```python
from build123d import *

# Parameters (mm, degrees)
CROQUIS1_W              = 60
CROQUIS1_H              = 65
SALIENTE_EXTRUIR1_DEPTH = 80
CROQUIS2_R              = 12.5
CROQUIS2_R_2            = 2
CROQUIS2_R_3            = 4
CORTAR_EXTRUIR1_DEPTH   = 120.268604419
CROQUIS3_W              = 38
CROQUIS3_H              = 70
CORTAR_EXTRUIR4_DEPTH   = 50
CROQUIS4_W              = 8.5
CROQUIS4_H              = 70
CORTAR_EXTRUIR5_DEPTH   = 120.268604419
CROQUIS6_R              = 12.5
CROQUIS6_R_2            = 2
CORTAR_EXTRUIR6_DEPTH   = 120.268604419
CROQUIS15_R             = 11
SALIENTE_EXTRUIR6_DEPTH = 0.1
CROQUIS16_R             = 10.5
CORTAR_EXTRUIR11_DEPTH  = 10
CORTAR_EXTRUIR12_REACH  = 116.175
CROQUIS17_R             = 7
CROQUIS10_W             = 23
CROQUIS10_H             = 35
CORTAR_EXTRUIR9_DEPTH   = 120.268604419
CROQUIS11_W             = 10
CROQUIS11_H             = 10
SALIENTE_EXTRUIR4_DEPTH = 10
SKETCH1_R               = 3.5
CUT_EXTRUDE1_DEPTH      = 113.805141727


with BuildPart() as part:
    # Croquis1 → Saliente-Extruir1 (new body)
    with BuildSketch(Plane(origin=(0, 0, 0), x_dir=(1, 0, 0), z_dir=(0, 1, 0))):
        with Locations((30, 32.5)):
            Rectangle(CROQUIS1_W, CROQUIS1_H)
    extrude(amount=SALIENTE_EXTRUIR1_DEPTH)

    # Croquis2 → Cortar-Extruir1 (cut, through all)
    with BuildSketch(Plane.ZY):
        with Locations((-35, 50)):
            Circle(CROQUIS2_R)
        with Locations((-50.5, 65.5)):
            Circle(CROQUIS2_R_2)
        with Locations((-19.5, 65.5)):
            Circle(CROQUIS2_R_2)
        with Locations((-19.5, 34.5)):
            Circle(CROQUIS2_R_2)
        with Locations((-50.5, 34.5)):
            Circle(CROQUIS2_R_2)
        with Locations((-60, 75)):
            Circle(CROQUIS2_R_3)
        with Locations((-10, 75)):
            Circle(CROQUIS2_R_3)
        with Locations((-10, 25)):
            Circle(CROQUIS2_R_3)
        with Locations((-60, 25)):
            Circle(CROQUIS2_R_3)
    extrude(amount=-CORTAR_EXTRUIR1_DEPTH, mode=Mode.SUBTRACT)

    # Croquis3 → Cortar-Extruir4 (cut)
    with BuildSketch(Plane(origin=(0, 0, -65), x_dir=(-1, 0, 0), z_dir=(0, 0, -1))):
        with Locations((-30, 35)):
            Rectangle(CROQUIS3_W, CROQUIS3_H)
    extrude(amount=-CORTAR_EXTRUIR4_DEPTH, mode=Mode.SUBTRACT)

    # Croquis4 → Cortar-Extruir5 (cut, through all)
    with BuildSketch(Plane.XY):
        with Locations((14.25, 35)):
            Rectangle(CROQUIS4_W, CROQUIS4_H)
        with Locations((45.75, 35)):
            Rectangle(CROQUIS4_W, CROQUIS4_H)
    extrude(amount=-CORTAR_EXTRUIR5_DEPTH, mode=Mode.SUBTRACT)

    # Croquis6 → Cortar-Extruir6 (cut, through all)
    with BuildSketch(Plane(origin=(0, 80, 0), x_dir=(1, 0, 0), z_dir=(0, 1, 0))):
        with Locations(Location((30, 35, 0), (0, 0, 270))):
            Circle(CROQUIS6_R)
        with Locations(Location((14.5, 50.5, 0), (0, 0, 270))):
            Circle(CROQUIS6_R_2)
        with Locations(Location((45.5, 50.5, 0), (0, 0, 270))):
            Circle(CROQUIS6_R_2)
        with Locations(Location((45.5, 19.5, 0), (0, 0, 270))):
            Circle(CROQUIS6_R_2)
        with Locations(Location((14.5, 19.5, 0), (0, 0, 270))):
            Circle(CROQUIS6_R_2)
    extrude(amount=-CORTAR_EXTRUIR6_DEPTH, mode=Mode.SUBTRACT)

    # Croquis15 → Saliente-Extruir6 (add)
    with BuildSketch(Plane.XY):
        with Locations(Location((30, 50, 0), (0, 0, 180))):
            Circle(CROQUIS15_R)
    extrude(amount=SALIENTE_EXTRUIR6_DEPTH)

    # Croquis16 → Cortar-Extruir11 (cut)
    with BuildSketch(Plane.XY.offset(0.1)):
        with Locations((30, 50)):
            Circle(CROQUIS16_R)
    extrude(amount=-CORTAR_EXTRUIR11_DEPTH, mode=Mode.SUBTRACT)

    # Croquis17 → Cortar-Extruir12 (cut, up to next)
    with BuildSketch(Plane.XY.offset(-9.9), mode=Mode.PRIVATE) as cortar_extruir12_sk1:
        with Locations((30, 50)):
            Circle(CROQUIS17_R)
    cortar_extruir12_tool1 = extrude(cortar_extruir12_sk1.sketch, amount=-CORTAR_EXTRUIR12_REACH, mode=Mode.PRIVATE) & part.part
    add(cortar_extruir12_tool1.solids().sort_by_distance((30, 50, -9.9))[0], mode=Mode.SUBTRACT)

    # Croquis10 → Cortar-Extruir9 (cut, through all)
    with BuildSketch(Plane.XY):
        with Locations((30, 17.5)):
            Rectangle(CROQUIS10_W, CROQUIS10_H)
    extrude(amount=-CORTAR_EXTRUIR9_DEPTH, mode=Mode.SUBTRACT)

    # Croquis11 → Saliente-Extruir4 (add)
    with BuildSketch(Plane.XY):
        with Locations((5, 5)):
            Rectangle(CROQUIS11_W, CROQUIS11_H)
        with Locations((55, 5)):
            Rectangle(CROQUIS11_W, CROQUIS11_H)
    saliente_extruir4 = extrude(amount=SALIENTE_EXTRUIR4_DEPTH)

    # Sketch1 → Cut-Extrude1 (cut, through all)
    with BuildSketch(Plane(origin=(0, 10, 0), x_dir=(1, 0, 0), z_dir=(0, 1, 0))):
        with Locations(Location((5, -5, 0), (0, 0, 270))):
            Circle(SKETCH1_R)
        with Locations(Location((55, -5, 0), (0, 0, 270))):
            Circle(SKETCH1_R)
    cut_extrude1 = extrude(amount=-CUT_EXTRUDE1_DEPTH, mode=Mode.SUBTRACT)

    # Mirror2: Saliente-Extruir4, Cut-Extrude1 across plane
    add(saliente_extruir4.mirror(Plane.XY.offset(-32.5)))
    add(cut_extrude1.mirror(Plane.XY.offset(-32.5)), mode=Mode.SUBTRACT)


solid = part.part
```
Can you work these out from the model? Positions are in its coordinate system, mm. A direction names the side the tool comes from. Give positions to 0.01 mm unless a question says otherwise; leave off trailing zeros. Write each loop counter-clockwise with the first axis right and the second up, starting at its lowest first coordinate (ties: lowest second). Pieces come first, ordered by that corner, then holes. Notation, with made-up numbers: (65.25, 61.25) -> (124.25, 61.25) arc R19 ccw to (124.25, 69.25) -> close; hole circle Ø5 at (-26.75, 81). An arc over 180 degrees is marked (long way). Write item = value, one per line.
(1) Suppose I cut it at A-A on x = 5. Count the separate pieces of the cut face and the enclosed holes in it, then the cut area to 3 significant figures.
Worked out:
separate_pieces = 3
enclosed_holes = 9
area = 4,520 mm^2
(2) Suppose I cut it at D-D on x = 45.5. Write out the boundary of the cut face in (y, z).
Worked out:
outline = (70, -65) -> (80, -65) -> (80, -52.5) -> (70, -52.5) -> close; (70, -48.5) -> (80, -48.5) -> (80, -21.5) -> (70, -21.5) -> close; (70, -17.5) -> (80, -17.5) -> (80, 0) -> (70, 0) -> close; hole circle Ø8 at (75, -60); hole circle Ø8 at (75, -10)
(3) For faces 5 (the face through (4.93, 67.483, -50.76)), 6 (the face through (9.6, 52.3, -65)), 7 (the face through (32, 43, -9.9)), which set-ups out of +Z, -Z, +X, -X, +Y, -Y let a thin tool reach every point of the face, with its end or its side?
Worked out:
face_5 = +X, -X
face_6 = -Z, +X, -X, +Y
face_7 = +Z
(4) I'm going to push flat-ended pins straight in: P1, Ø20, axis at y = 50, z = -35, coming from the -X side; P2, Ø4.5, axis at x = 45.5, z = -50.5, coming from the +Y side; P3, Ø6.5, axis at x = 34, y = 45.5, coming from the +Z side; P4, Ø16.5, axis at x = 26, z = -7.5, coming from the -Y side. Where does each tip first touch, or does it pass through?
Worked out:
P1 = through
P2 = 80
P3 = -9.9
P4 = 35
(5) I need wall thicknesses on probe 1 along X at (y, z) = (24, -24.5); probe 2 along Y at (x, z) = (57, -60); probe 3 along Y at (x, z) = (25, -10). Which ranges of each line are inside material? Lowest first, please. Write a range as from..to.
Worked out:
probe_1 = 0..10, 50..60
probe_2 = 0..21, 29..71, 79..80
probe_3 = 35..45.1, 54.9..71, 79..80
(6) Thinking about a two-plate mould opening in Z: for faces 1 (the face through (43.548, 75.07, -50.934)), 2 (the face through (33, 57, -15)), 3 (the face through (50, 35, -32)), 4 (the face through (54.93, 67.483, -19.76)), which applies, released by +Z, released by -Z, zero draft, split by the parting line, or undercut?
Worked out:
face_1 = undercut
face_2 = released by -Z
face_3 = zero draft
face_4 = undercut
(7) Suppose I cut it at B-B on z = -60. Write out the boundary of the cut face in (x, y).
Worked out:
outline = (0, 0) -> (10, 0) -> (10, 21) -> (0, 21) -> close; (0, 29) -> (10, 29) -> (10, 70) -> (50, 70) -> (50, 29) -> (60, 29) -> (60, 71) -> (0, 71) -> close; (0, 79) -> (60, 79) -> (60, 80) -> (0, 80) -> close; (50, 0) -> (60, 0) -> (60, 21) -> (50, 21) -> close
